Could you check a few things on this model? Use its own coordinates, in mm. A direction names the side the tool comes from. Give positions to 0.01 mm unless a question says otherwise; leave off trailing zeros. Loops run counter-clockwise (first coordinate to the right, second up) from the corner with the lowest first, then second, coordinate; pieces in that order, holes last. Notation, with made-up numbers: (36.25, 59.25) - (88.25, 59.25) arc R32 ccw to (88.25, 97.25) - close; hole circle Ø5 at (18.5, 76.5). An arc over 180 degrees is marked (long way). Use CSV: the item, a comma, the result in double quotes.
Autodesk Inventor part; units mm, degrees
ref_plane "YZ Plane" through (0, 0, 0) normal (1, 0, 0) x (0, 1, 0)
ref_plane "XZ Plane" through (0, 0, 0) normal (0, 1, 0) x (-1, 0, 0)
ref_plane "XY Plane" through (0, 0, 0) normal (0, 0, 1) x (1, 0, 0)
sketch "Sketch1" plane through (0, 0, 0) normal (1, 0, 0) x (0, 1, 0)
  circle A0 centre (0, 0) radius 5.0038
  circle A1 centre (0, 0) radius 4.0005
  dimension "d0" = 10.0076
  dimension "d1" = 8.001
extrude "Extrusion1" add sketch "Sketch1" along normal blind 11.5062
sketch "Sketch2" plane through (11.5062, 0, 0) normal (1, 0, 0) x (0, 0, -1)
  circle A0 centre (0, 0) radius 12.7
  circle A1 centre (0, 0) radius 4.0005
  dimension "d4" = 25.4
  dimension "d7" = 8.001
extrude "Extrusion2" add sketch "Sketch2" along normal blind 15.6464
chamfer "Chamfer1" distance 0.254 angle 45 3 edges at (0, -5.0038, 0) (11.5062, 0, 12.7) (27.1526, 0, 12.7)
properties part number "Flex_Bushing"
1) I'm going to push flat-ended pins straight in: P1, Ø12, axis at x = 13, z = 8, coming from the -Y side; P2, Ø3, axis at y = -2, z = 6, coming from the -X side; P3, Ø6, axis at x = 23.5, z = -9.5, coming from the +Y side. Where does each tip first touch, or does it pass through?
Answer below:
P1,"stops at y = -12.54"
P2,"stops at x = 0.07"
P3,"stops at y = 10.91"
2) We'd pull the mould along Y, two halves only. Please class faces 3 (the cylindrical face through (13.39, -2.11, -3.4)), 4 (the cylindrical face through (19.22, 12.4, 2.75)), 5 (the flat face through (0, -4, -2)): +Y half, -Y half, draft (parallel to the pull), parting line (faces both ways), or undercut.
Answer below:
face 3,"undercut"
face 4,"parting line"
face 5,"draft"
3) Which directions (+Z, -Z, +X, -X, +Y, -Y) give clear straight access to the entire face, cutting with the end or side of a thin tool? Please do faces 1 (the flat face through (27.153, 3, 3)), 2 (the flat face through (11.506, 0.2, -5.4)).
Answer below:
face 1,"+Z, -Z, +X, +Y, -Y"
face 2,"-X"
4) I need wall thicknesses on line 1 along Y through (x, z) = (13.75, 0); line 2 along Z through (x, y) = (10.75, 0); line 3 along X through (y, z) = (10.75, 3.5). Which ranges of each line are inside material? Lowest first, please.
Answer below:
line 1,"y = -12.7 to -4, 4 to 12.7"
line 2,"z = -5 to -4, 4 to 5"
line 3,"x = 11.51 to 27.15"
5) Suppose I cut it at A-A (z = 0). Please give me the cut outline in (x, y), plus the area to 3 significant figures.
Answer below:
outline,"(0, -4.75) - (0.25, -5) - (11.51, -5) - (11.51, -12.45) - (11.76, -12.7) - (26.9, -12.7) - (27.15, -12.45) - (27.15, -4) - (0, -4) - close; (0, 4) - (27.15, 4) - (27.15, 12.45) - (26.9, 12.7) - (11.76, 12.7) - (11.51, 12.45) - (11.51, 5) - (0.25, 5) - (0, 4.75) - close"
area,"295 mm2"
